from build123d import *

# Parameters (mm, degrees)
F0_W         = 30
F0_H         = 30
F1_DEPTH     = 20
F2_W         = 25.9800008498
F2_H         = 25.9800008498
F3_DEPTH     = 2.5
F4_W         = 25.9800008498
F4_H         = 25.9800008498
F5_DEPTH     = 2.5
F6_R         = 5
F7_T         = 2.5
F7_T3_DEPTH  = 20.9800008498
F7_T5_DEPTH  = 20.9800008498
F7_T8_ANGLE  = 90.000000001
F7_T10_ANGLE = 90.000000001
F7_T12_ANGLE = 90.000000001
F7_T14_ANGLE = 90.000000001
F8_R         = 1.4393768416
F9_DEPTH     = 25


# Not quite as in the source:
# - a shell that OpenCascade refuses in one call is made with other operations: the cavity is built on its own and cut out


with BuildPart() as f1:
    # F0 (on Top) → F1 (new body)
    with BuildSketch(Plane.XY):
        Rectangle(F0_W, F0_H)
    extrude(amount=F1_DEPTH)

    # F2 (on face) → F3 (cut)
    with BuildSketch(Plane.XY):
        Rectangle(F2_W, F2_H)
    extrude(amount=F3_DEPTH, mode=Mode.SUBTRACT)

    # F4 (on face) → F5 (cut)
    with BuildSketch(Plane.XY.offset(20)):
        Rectangle(F4_W, F4_H)
    extrude(amount=-F5_DEPTH, mode=Mode.SUBTRACT)

    # F6
    f6_edges = [f1.edges().sort_by_distance(p)[0] for p in [
        (-15, -15, 10),
        (-12.99, -12.99, 18.75),
        (-12.99, 12.99, 18.75),
        (12.99, -12.99, 18.75),
        (15, -15, 10),
        (15, 15, 10),
        (-15, 15, 10),
        (12.99, 12.99, 18.75),
        (-12.99, 12.99, 1.25),
        (12.99, -12.99, 1.25),
        (-12.99, -12.99, 1.25),
        (12.99, 12.99, 1.25),
    ]]
    fillet(f6_edges, radius=F6_R)

    # F7: shell of thickness 2.5, made by hand


with BuildPart() as f7_core1:
    # F7_t2: copy of F1
    add(f1.part)

    # the walls: a layer under each face that stays
    f7_faces = [f7_core1.faces().sort_by_distance(p)[0] for p in [
        (0, 15, 10),
        (-12.8571428571, -12.8571428571, 0),
        (13.5355339059, 13.5355339059, 10),
        (-13.5355339059, 13.5355339059, 10),
        (-12.8571428571, -12.8571428571, 20),
        (15, 0, 10),
        (-15, 0, 10),
        (13.5355339059, -13.5355339059, 10),
        (-13.5355339059, -13.5355339059, 10),
        (0, -15, 10),
        (-12.9900004249, 0, 1.25),
        (-11.5255343308, 11.5255343308, 1.25),
        (-11.5255343308, -11.5255343308, 1.25),
        (0, 12.9900004249, 1.25),
        (0, -12.9900004249, 1.25),
        (11.5255343308, 11.5255343308, 1.25),
        (11.5255343308, -11.5255343308, 1.25),
        (12.9900004249, 0, 1.25),
        (0, 12.9900004249, 18.75),
        (11.5255343308, 11.5255343308, 18.75),
        (-11.5255343308, 11.5255343308, 18.75),
        (12.9900004249, 0, 18.75),
        (-12.9900004249, 0, 18.75),
        (11.5255343308, -11.5255343308, 18.75),
        (-11.5255343308, -11.5255343308, 18.75),
        (0, -12.9900004249, 18.75),
        (0, 0, 2.5),
    ]]
    thicken(f7_faces, amount=-F7_T, mode=Mode.SUBTRACT)

    # F7_s4 → F7_t3 (cut)
    with BuildSketch(Plane.XZ.offset(-10.4900004249)):
        Polygon((-12.9650004249, 2.475), (-15.4900004249, 2.5), (-15.4900004249, 5), (-12.9900004249, 5), align=None)
        Polygon((12.9650004249, 2.475), (15.4900004249, 2.5), (15.4900004249, 5), (12.9900004249, 5), align=None)
    extrude(amount=F7_T3_DEPTH, mode=Mode.SUBTRACT)

    # F7_s6 → F7_t5 (cut)
    with BuildSketch(Plane.YZ.offset(-10.4900004249)):
        Polygon((12.9650004249, 2.475), (15.4900004249, 2.5), (15.4900004249, 5), (12.9900004249, 5), align=None)
        Polygon((-12.9650004249, 2.475), (-15.4900004249, 2.5), (-15.4900004249, 5), (-12.9900004249, 5), align=None)
    extrude(amount=F7_T5_DEPTH, mode=Mode.SUBTRACT)

    # F7_s7 → F7_t8 (revolve, cut)
    with BuildSketch(Plane.XZ.offset(-7.9900004249)):
        Polygon((-12.9650004249, 2.475), (-15.4900004249, 2.5), (-15.4900004249, 5), (-12.9900004249, 5), align=None)
    revolve(axis=Axis((-7.9900004249, 7.9900004249, 2.5), (0, 0, -1)), revolution_arc=F7_T8_ANGLE, mode=Mode.SUBTRACT)

    # F7_s9 → F7_t10 (revolve, cut)
    with BuildSketch(Plane.XZ.offset(7.9900004249)):
        Polygon((-12.9650004249, 2.475), (-15.4900004249, 2.5), (-15.4900004249, 5), (-12.9900004249, 5), align=None)
    revolve(axis=Axis((-7.9900004249, -7.9900004249, 2.5), (0, 0, 1)), revolution_arc=F7_T10_ANGLE, mode=Mode.SUBTRACT)

    # F7_s11 → F7_t12 (revolve, cut)
    with BuildSketch(Plane.XZ.offset(-7.9900004249)):
        Polygon((12.9650004249, 2.475), (15.4900004249, 2.5), (15.4900004249, 5), (12.9900004249, 5), align=None)
    revolve(axis=Axis((7.9900004249, 7.9900004249, 2.5), (0, 0, 1)), revolution_arc=F7_T12_ANGLE, mode=Mode.SUBTRACT)

    # F7_s13 → F7_t14 (revolve, cut)
    with BuildSketch(Plane.YZ.offset(7.9900004249)):
        Polygon((-12.9650004249, 2.475), (-15.4900004249, 2.5), (-15.4900004249, 5), (-12.9900004249, 5), align=None)
    revolve(axis=Axis((7.9900004249, -7.9900004249, 2.5), (0, 0, 1)), revolution_arc=F7_T14_ANGLE, mode=Mode.SUBTRACT)


with BuildPart() as f1_1:
    add(f1.part)

    # what is left inside the walls is the cavity
    f7_cavity = [f7_core1.part.solids().sort_by_distance(p)[0] for p in [
        (0, -4.166667, 17.475),
    ]]
    add(f7_cavity, mode=Mode.SUBTRACT)

    # F8 (on face) → F9 (cut)
    with BuildSketch(Plane.XY.offset(5)):
        Circle(F8_R)
        with Locations((0, 7.2)):
            Circle(F8_R)
        with Locations((5.1, 0)):
            Circle(F8_R)
        with Locations((5.1, 7.2)):
            Circle(F8_R)
        with Locations((10.2, 0)):
            Circle(F8_R)
        with Locations((10.2, 7.2)):
            Circle(F8_R)
        with Locations((-5.1, 0)):
            Circle(F8_R)
        with Locations((-10.2, 0)):
            Circle(F8_R)
        with Locations((-10.2, 7.2)):
            Circle(F8_R)
        with Locations((-5.1, 7.2)):
            Circle(F8_R)
    extrude(amount=-F9_DEPTH, mode=Mode.SUBTRACT)


solid = f1_1.part
Can you work these out from the model? Positions are in its coordinate system, mm. A direction names the side the tool comes from. Coordinates: 2 decimals unless noted, no trailing zeros. Write each loop counter-clockwise with the first axis right and the second up, starting at its lowest first coordinate (ties: lowest second). Pieces come first, ordered by that corner, then holes.
Q1. Please list where these lines run through material, in increasing order: L1, parallel to Y at x = 5.1, z = 3.6; L2, parallel to X at y = 3.75, z = 15; L3, parallel to X at y = -4, z = 1.
Results found:
L1: y = -15 to -1.44, 1.44 to 5.76, 8.64 to 15
L2: x = -15 to -12.5, 12.5 to 15
L3: x = -15 to -12.99, 12.99 to 15
Q2. If we mould it in two halves opening along X, with no side actions, what happens to faces 1 (the face through (0, -3, 2.5)), 2 (the face through (0, -15, 10)), 3 (the face through (-14, -13, 10))? For each: +X half, -X half, draft (parallel to the pull), parting line (faces both ways), or undercut.
Results found:
face 1: undercut
face 2: draft
face 3: -X half
Q3. Which directions (+Z, -Z, +X, -X, +Y, -Y) give clear straight access to the entire face, cutting with the end or side of a thin tool? Please do faces 4 (the face through (-11.7, 11.6, 17.5)), 5 (the face through (-12.99, 0, 1)), 6 (the face through (11.56, 11.49, 18.73)), 7 (the face through (15, 0, 10)).
Results found:
face 4: none
face 5: -Z
face 6: +Z
face 7: +Z, -Z, +X, +Y, -Y
Q4. Imagine slicing it at B-B, the plane z = 8.75. List the corners of the cut face in (x, y) for me, plus the area to 3 significant figures.
Results found:
outline: (-15, -10) arc R5 ccw to (-10, -15) - (10, -15) arc R5 ccw to (15, -10) - (15, 10) arc R5 ccw to (10, 15) - (-10, 15) arc R5 ccw to (-15, 10) - close; hole (-12.5, -10) arc R2.5 ccw to (-10, -12.5) - (10, -12.5) arc R2.5 ccw to (12.5, -10) - (12.5, 10) arc R2.5 ccw to (10, 12.5) - (-10, 12.5) arc R2.5 ccw to (-12.5, 10) - close
area: 259 mm2
Q5. Imagine slicing it at A-A, the plane x = 5.1. List the corners of the cut face in (y, z) for me.
Results found:
outline: (-15, 0) - (-12.99, 0) - (-12.99, 2.5) - (-1.44, 2.5) - (-1.44, 5) - (-12.5, 5) - (-12.5, 17.5) - (-12.99, 17.5) - (-12.99, 20) - (-15, 20) - close; (1.44, 2.5) - (5.76, 2.5) - (5.76, 5) - (1.44, 5) - close; (8.64, 2.5) - (12.99, 2.5) - (12.99, 0) - (15, 0) - (15, 20) - (12.99, 20) - (12.99, 17.5) - (12.5, 17.5) - (12.5, 5) - (8.64, 5) - close
Q6. Imagine slicing it at D-D, the plane y = 11.25. List the corners of the cut face in (x, z) for me, plus the area to 3 significant figures.
Results found:
outline: (-14.84, 0) - (-11.78, 0) - (-11.78, 2.5) - (11.78, 2.5) - (11.78, 0) - (14.84, 0) - (14.84, 20) - (11.78, 20) - (11.78, 17.5) - (12.17, 17.5) - (12.17, 5) - (-12.17, 5) - (-12.17, 17.5) - (-11.78, 17.5) - (-11.78, 20) - (-14.84, 20) - close
area: 172 mm2
Q7. For P1, Ø1.2, axis at x = -12, y = -11, coming from the -Z side; P2, Ø3.5, axis at x = -5.1, y = 7.2, coming from the +Z side; P3, Ø0.7, axis at x = -11, y = 11, coming from the -Z side, each with a flat end and sliding along its axis, tell me the tip position at first contact or that it passes through.
Results found:
P1: stops at z = 0
P2: stops at z = 5
P3: stops at z = 2.5
Q8. Imagine slicing it at C-C, the plane y = 7.2. Count the separate pieces of the cut face and the enclosed holes in it, plus the area to 3 significant figures.
Results found:
separate pieces: 6
enclosed holes: 0
area: 122 mm2
